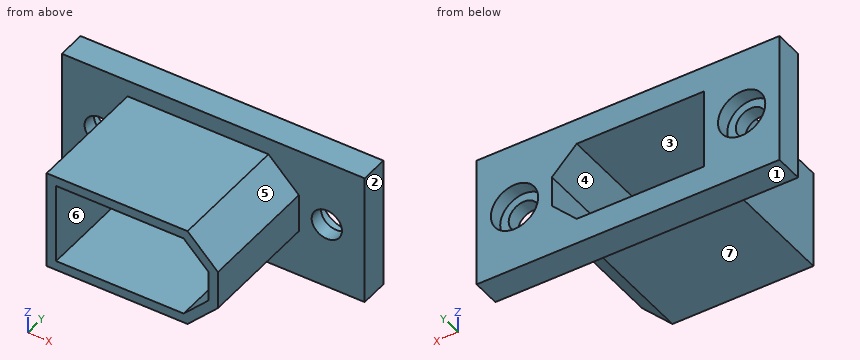
```python
from build123d import *

# Parameters (mm, degrees)
SKETCH1_W           = 32
SKETCH1_H           = 14
BOSS_EXTRUDE1_DEPTH = 3
CUT_EXTRUDE1_DEPTH  = 3
BOSS_EXTRUDE2_DEPTH = 16
SKETCH4_R           = 1.6
CUT_EXTRUDE2_DEPTH  = 3
SKETCH5_R           = 2.5
CUT_EXTRUDE3_DEPTH  = 1.5


with BuildPart() as part:
    # Sketch1 → Boss-Extrude1 (new body)
    with BuildSketch(Plane(origin=(0, 0, 0), x_dir=(1, 0, 0), z_dir=(0, 1, 0))):
        Rectangle(SKETCH1_W, SKETCH1_H)
    extrude(amount=BOSS_EXTRUDE1_DEPTH)

    # Sketch2 → Cut-Extrude1 (cut)
    with BuildSketch(Plane(origin=(0, 3, 0), x_dir=(1, 0, 0), z_dir=(0, 1, 0))):
        Polygon((5.424264069, -4.25), (-8.05, -4.25), (-8.05, 4.25), (5.424264069, 4.25), (8.05, 1.624264069), (8.05, -1.624264069), align=None)
    extrude(amount=-CUT_EXTRUDE1_DEPTH, mode=Mode.SUBTRACT)

    # Sketch3 → Boss-Extrude2 (add)
    with BuildSketch(Plane(origin=(0, 3, 0), x_dir=(1, 0, 0), z_dir=(0, 1, 0))):
        Polygon((5.838477631, -5.25), (-9.05, -5.25), (-9.05, 5.25), (5.838477631, 5.25), (9.05, 2.038477631), (9.05, -2.038477631), align=None)
        Polygon((-8.05, -4.25), (-8.05, 4.25), (5.424264069, 4.25), (8.05, 1.624264069), (8.05, -1.624264069), (5.424264069, -4.25), align=None, mode=Mode.SUBTRACT)
    extrude(amount=-BOSS_EXTRUDE2_DEPTH)

    # Sketch4 → Cut-Extrude2 (cut)
    with BuildSketch(Plane(origin=(0, 3, 0), x_dir=(1, 0, 0), z_dir=(0, 1, 0))):
        with Locations(Location((-12, 0, 0), (0, 0, 270))):
            Circle(SKETCH4_R)
        with Locations(Location((12, 0, 0), (0, 0, 270))):
            Circle(SKETCH4_R)
    extrude(amount=-CUT_EXTRUDE2_DEPTH, mode=Mode.SUBTRACT)

    # Sketch5 → Cut-Extrude3 (cut)
    with BuildSketch(Plane(origin=(0, 3, 0), x_dir=(1, 0, 0), z_dir=(0, 1, 0))):
        with Locations(Location((-12, 0, 0), (0, 0, 270))):
            Circle(SKETCH5_R)
        with Locations(Location((12, 0, 0), (0, 0, 270))):
            Circle(SKETCH5_R)
    extrude(amount=-CUT_EXTRUDE3_DEPTH, mode=Mode.SUBTRACT)


solid = part.part
```
Part model, mm, in its own coordinate system. Face numbers are marked on the shaded views. A direction names the side the tool comes from. Give positions to 0.01 mm unless a question says otherwise; leave off trailing zeros. Loops run counter-clockwise (first coordinate to the right, second up) from the corner with the lowest first, then second, coordinate; pieces in that order, holes last. Notation, with made-up numbers: M -24.5,20 L -7.5,20 A15 cw -7.5,44 Z; hole C 45.5,-3.75 d2. An arc over 180 degrees is marked long. Return JSON: item names as keys, results as strings.
1) Saw through at D-D, the plane x = -3. List the corners of the cut face in (y, z), then the cut area to 3 significant figures.
Calculated:
{"outline": "M -13,-5.25 L 0,-5.25 L 0,-7 L 3,-7 L 3,-4.25 L -13,-4.25 Z; M -13,4.25 L 3,4.25 L 3,7 L 0,7 L 0,5.25 L -13,5.25 Z", "area": "42.5 mm2"}
2) 3-axis set-ups, long thin cutter, end or side, ignore diameter. For the marked faces 5, 6 and 7: which of +Z, -Z, +X, -X, +Y, -Y reach the whole face in a straight line?
Calculated:
{"face 5": "+Z, +X, -Y", "face 6": "+Y, -Y", "face 7": "-Z, +X, -X, -Y"}
3) Drill centre lines: line 1 (X direction, y = 2.65, z = 0); line 2 (X direction, y = 0.65, z = 0); line 3 (Z direction, x = -4.5, y = -4.5). Where is each one in solid material? Low to high.
Calculated:
{"line 1": "x = -16 to -14.5, -9.5 to -8.05, 8.05 to 9.5, 14.5 to 16", "line 2": "x = -16 to -13.6, -10.4 to -8.05, 8.05 to 10.4, 13.6 to 16", "line 3": "z = -5.25 to -4.25, 4.25 to 5.25"}
4) Pull direction Z, two halves, no side cores. Call the marked faces 1, 2, 3 and 4: released by +Z, released by -Z, zero draft, split by the parting line, or undercut.
Calculated:
{"face 1": "released by -Z", "face 2": "zero draft", "face 3": "undercut", "face 4": "undercut"}
5) Saw through at A-A, the plane z = 0. List the corners of the cut face in (x, y), then the cut area to 3 significant figures.
Calculated:
{"outline": "M -16,0 L -13.6,0 L -13.6,1.5 L -14.5,1.5 L -14.5,3 L -16,3 Z; M -10.4,0 L -9.05,0 L -9.05,-13 L -8.05,-13 L -8.05,3 L -9.5,3 L -9.5,1.5 L -10.4,1.5 Z; M 8.05,-13 L 9.05,-13 L 9.05,0 L 10.4,0 L 10.4,1.5 L 9.5,1.5 L 9.5,3 L 8.05,3 Z; M 13.6,0 L 16,0 L 16,3 L 14.5,3 L 14.5,1.5 L 13.6,1.5 Z", "area": "49.1 mm2"}
6) Flat gauge pins, fed straight in: pin 1 Ø2.5 at (x, z) = (-12, 0) entering from -Y; pin 2 Ø6.5 at (x, y) = (-2.5, -8) entering from +Z; pin 3 Ø4 at (x, z) = (12, 0) entering from +Y; pin 4 Ø1.6 at (y, z) = (-2, -0.5) entering from -X. Where does each tip first touch, or does it go through?
Calculated:
{"pin 1": "passes through", "pin 2": "stops at z = 5.25", "pin 3": "stops at y = 1.5", "pin 4": "stops at x = -9.05"}
7) Saw through at B-B, the plane x = 12. List the corners of the cut face in (y, z).
Calculated:
{"outline": "M 0,-7 L 3,-7 L 3,-2.5 L 1.5,-2.5 L 1.5,-1.6 L 0,-1.6 Z; M 0,1.6 L 1.5,1.6 L 1.5,2.5 L 3,2.5 L 3,7 L 0,7 Z"}
8) Saw through at C-C, the plane y = -2. List the corners of the cut face in (x, z).
Calculated:
{"outline": "M -9.05,-5.25 L 5.84,-5.25 L 9.05,-2.04 L 9.05,2.04 L 5.84,5.25 L -9.05,5.25 Z; hole M -8.05,-4.25 L 5.42,-4.25 L 8.05,-1.62 L 8.05,1.62 L 5.42,4.25 L -8.05,4.25 Z"}
